```python
from build123d import *

# Parameters (mm, degrees)
SKETCH1_W           = 6.023507921
SKETCH1_H           = 9
SKETCH1_W_2         = 6
SKETCH1_H_2         = 6
SKETCH1_H_3         = 12
BOSS_EXTRUDE1_DEPTH = 6


with BuildPart() as part:
    # Sketch1 → Boss-Extrude1 (new body)
    with BuildSketch(Plane(origin=(0, 0, 0), x_dir=(1, 0, 0), z_dir=(0, 1, 0))):
        Polygon((-30.457136098, 33.379680679), (-54.770597518, 33.379680679), (-54.770597518, -45.488511926), (-24.197851339, -45.488511926), (-24.197851339, -48.488511926), (-18.197851339, -48.488511926), (-18.197851339, -45.488511926), (-12.197851339, -45.488511926), (-12.197851339, -51.488511926), (12.197851339, -51.488511926), (12.197851339, -45.488511926), (18.197851339, -45.488511926), (18.197851339, -48.488511926), (24.197851339, -48.488511926), (24.197851339, -45.488511926), (54.723581676, -45.488511926), (54.723581676, 33.379680679), (30.410120257, 33.379680679), (30.410120257, 27.379680679), (12.410120257, 27.379680679), (12.410120257, 33.379680679), (-12.457136098, 33.379680679), (-12.457136098, 27.379680679), (-30.457136098, 27.379680679), align=None)
        with Locations((-45.385335637, -33.07427073)):
            Rectangle(SKETCH1_W, SKETCH1_H, mode=Mode.SUBTRACT)
        with Locations((-15.197851339, -36.488511926)):
            Rectangle(SKETCH1_W_2, SKETCH1_H_2, mode=Mode.SUBTRACT)
        with Locations((-39.373581676, -21.614283631)):
            Rectangle(SKETCH1_W_2, SKETCH1_H_3, mode=Mode.SUBTRACT)
        with Locations((15.197851339, -36.488511926)):
            Rectangle(SKETCH1_W_2, SKETCH1_H_2, mode=Mode.SUBTRACT)
        with Locations((45.373581676, -33.07427073)):
            Rectangle(SKETCH1_W_2, SKETCH1_H, mode=Mode.SUBTRACT)
        with Locations((39.373581676, -21.614283631)):
            Rectangle(SKETCH1_W_2, SKETCH1_H_3, mode=Mode.SUBTRACT)
        Polygon((-36.373581676, 2.385716369), (-42.373581676, 2.385716369), (-42.373581676, 5.42572927), (-48.397089597, 5.42572927), (-48.397089597, 20.42572927), (-42.397089597, 20.42572927), (-42.397089597, 14.385716369), (-36.373581676, 14.385716369), align=None, mode=Mode.SUBTRACT)
        with BuildLine():
            Line((-12.587492722, 13.293717765), (-7.349609214, 22.548897144))
            Line((-7.349609214, 22.548897144), (7.326101293, 22.548897144))
            Line((7.326101293, 22.548897144), (12.578685825, 13.267741508))
            ThreePointArc((12.578685825, 13.267741508), (18.679992808, 16.942587364), (23.291850895, 11.51476976))
            ThreePointArc((23.291850895, 11.51476976), (22.796616824, 9.23391071), (21.400098894, 7.363800429))
            Line((21.400098894, 7.363800429), (31.116785699, 7.363800429))
            Line((31.116785699, 7.363800429), (31.116785699, -19.488511926))
            Line((31.116785699, -19.488511926), (18.197851339, -19.488511926))
            Line((18.197851339, -19.488511926), (18.197851339, -25.488511926))
            Line((18.197851339, -25.488511926), (12.197851339, -25.488511926))
            Line((12.197851339, -25.488511926), (12.197851339, -22.488511926))
            Line((12.197851339, -22.488511926), (-12.197851339, -22.488511926))
            Line((-12.197851339, -22.488511926), (-12.197851339, -25.488511926))
            Line((-12.197851339, -25.488511926), (-18.221359259, -25.488511926))
            Line((-18.221359259, -25.488511926), (-18.221359259, -19.488511926))
            Line((-18.221359259, -19.488511926), (-31.140293619, -19.488511926))
            Line((-31.140293619, -19.488511926), (-31.140293619, 7.363800429))
            Line((-31.140293619, 7.363800429), (-21.400098894, 7.363800429))
            ThreePointArc((-21.400098894, 7.363800429), (-20.862334868, 16.077896777), (-12.587492722, 13.293717765))
        make_face(mode=Mode.SUBTRACT)
        Polygon((42.373581676, 2.385716369), (36.373581676, 2.385716369), (36.373581676, 14.385716369), (42.373581676, 14.385716369), (42.373581676, 20.42572927), (48.373581676, 20.42572927), (48.373581676, 5.42572927), (42.373581676, 5.42572927), align=None, mode=Mode.SUBTRACT)
    extrude(amount=BOSS_EXTRUDE1_DEPTH)


solid = part.part
```
Design review of the part built by this model. Coordinates are the model's own, in mm. A direction names the side the tool comes from. Coordinates: 2 decimals unless noted, no trailing zeros. Order: outer loops, then holes, each group sorted by start corner. A loop starts at its lowest first (then second) coordinate and runs counter-clockwise, first axis right, second up.
1) Mouldability with a two-part tool opening along X and no side actions: class faces 1 (the flat face through (-45, 3, 28.574)), 2 (the flat face through (43, 3, -33.38)) as +X half, -X half, draft (parallel to the pull), parting line (faces both ways), or undercut.
2) For faces 3 (the flat face through (-12.198, 3, 48)), 4 (the flat face through (15, 3, 25.489)), 5 (the flat face through (-12.457, 3, -30)), list the 3-axis set-ups (+Z, -Z, +X, -X, +Y, -Y) from which the entire face can be reached by the end or side of a thin tool; tool diameter is ignored.
3) Take a section at A-A, the plane x = 43.5. Give the boundary of the cut face in (y, z).
4) Clearance check with a flat-ended pin moving along its axis: pin 1 (1.8 mm diameter, centred on x = 46.5, y = 4, fed in from +Z). State where the tip first meets the part, or that it passes through.
5) Wall thickness on line 1 along X through (y, z) = (0.6, -27.5); line 2 along X through (y, z) = (5.7, 33); line 3 along X through (y, z) = (4.8, 37.5): over which ranges is each line inside the solid? List them lowest first.
6) Take a section at C-C, the plane y = 1.6. State how many separate pieces and enclosed holes the cut face has, and give its area (3 significant figures).
7) Take a section at B-B, the plane z = 18. Give the boundary of the cut face in (x, y), and give its area (3 significant figures).
Returned:
1. face 1: undercut
1. face 2: draft
2. face 3: +Z, +Y, -Y
2. face 4: +Y, -Y
2. face 5: -Z, +Y, -Y
3. outline: (0, -33.38) - (6, -33.38) - (6, -20.43) - (0, -20.43) - close; (0, -5.43) - (6, -5.43) - (6, 28.57) - (0, 28.57) - close; (0, 37.57) - (6, 37.57) - (6, 45.49) - (0, 45.49) - close
4. pin 1: stops at z = 45.49
5. line 1: x = -54.77 to -30.46, -12.46 to 12.41, 30.41 to 54.72
5. line 2: x = -54.77 to -48.4, -42.37 to 42.37, 48.37 to 54.72
5. line 3: x = -54.77 to -48.4, -42.37 to -18.2, -12.2 to 12.2, 18.2 to 42.37, 48.37 to 54.72
6. separate pieces: 1
6. enclosed holes: 9
6. area: 5,620 mm2
7. outline: (-54.77, 0) - (-42.37, 0) - (-42.37, 6) - (-54.77, 6) - close; (-36.37, 0) - (-31.14, 0) - (-31.14, 6) - (-36.37, 6) - close; (31.12, 0) - (36.37, 0) - (36.37, 6) - (31.12, 6) - close; (42.37, 0) - (54.72, 0) - (54.72, 6) - (42.37, 6) - close
7. area: 211 mm2
